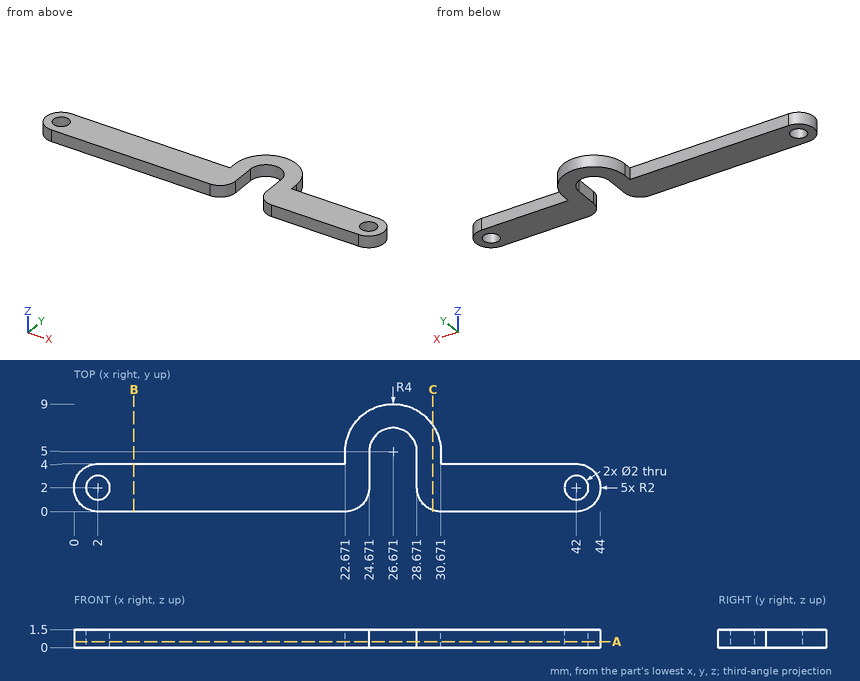
Part print with two shaded views. Sizes in mm from the minimum x, y, z corner. Round coordinates to 2 decimals unless told otherwise and drop trailing zeros. Write each loop counter-clockwise with the first axis right and the second up, starting at its lowest first coordinate (ties: lowest second). Pieces come first, ordered by that corner, then holes. Notation, with made-up numbers: (31.25, 82.25) -> (46.25, 82.25) arc R12 cw to (46.25, 88.25) -> close; hole circle Ø7 at (0.5, -8). An arc over 180 degrees is marked (long way). Put each result on its own line as item: value.
Item 1: Wall check: probe 1 along X at (y, z) = (1.25, 0.55) (1 decimal); probe 2 along X at (y, z) = (4.75, 0.6); probe 3 along X at (y, z) = (1.5, 1.25) (1 decimal). Give the ranges that are in metal, low to high. Write a range as from..to.
Here are the results:
probe 1: x = 0.1..1.3, 2.7..24.5, 28.8..41.3, 42.7..43.9
probe 2: x = 22.67..24.67, 28.67..30.67
probe 3: x = 0.1..1.1, 2.9..24.6, 28.7..41.1, 42.9..43.9
Item 2: Slice it at C-C, the plane x = 30. Give the cut face in (y, z).
Here are the results:
outline: (0.12, 0) -> (7.22, 0) -> (7.22, 1.5) -> (0.12, 1.5) -> close
Item 3: Flat gauge pins, fed straight in: P1, Ø0.8, axis at x = 11, z = 0.5, coming from the +Y side; P2, Ø0.8, axis at y = 3.5, z = 1, coming from the -X side; P3, Ø0.8, axis at y = 4.5, z = 1, coming from the -X side. Where does each tip first touch, or does it go through?
Here are the results:
P1: stops at y = 4
P2: stops at x = 0.33
P3: stops at x = 22.67
Item 4: Slice it at A-A, the plane z = 0.5. Give the cut face in (x, y).
Here are the results:
outline: (2, 0) -> (22.67, 0) arc R2 ccw to (24.67, 2) -> (24.67, 5) arc R2 cw to (28.67, 5) -> (28.67, 2) arc R2 ccw to (30.67, 0) -> (42, 0) arc R2 ccw to (42, 4) -> (30.67, 4) -> (30.67, 5) arc R4 ccw to (22.67, 5) -> (22.67, 4) -> (2, 4) arc R2 ccw to start; hole circle Ø2 at (2, 2); hole circle Ø2 at (42, 2)
Item 5: Slice it at B-B, the plane x = 5. Give the cut face in (y, z).
Here are the results:
outline: (0, 0) -> (4, 0) -> (4, 1.5) -> (0, 1.5) -> close
